```python
from build123d import *

# Parameters (mm, degrees)
F1_DEPTH = 25.4
F2_R     = 51.507819
F3_DEPTH = 203.2
F5_DEPTH = 25.4


with BuildPart() as f1:
    # F0 (on Front) → F1 (new body)
    with BuildSketch(Plane.XZ):
        Polygon((-28.796132, -69.520012), (28.796132, -69.520012), (69.520012, -28.796132), (69.520012, 28.796132), (28.796132, 69.520012), (-28.796132, 69.520012), (-69.520012, 28.796132), (-69.520012, -28.796132), align=None)
    extrude(amount=F1_DEPTH)

    # F2 (on Front) → F3 (join)
    with BuildSketch(Plane.XZ):
        Circle(F2_R)
    extrude(amount=F3_DEPTH)

    # F4 (on face) → F5 (join)
    with BuildSketch(Plane.XZ.offset(25.4)):
        Polygon((-28.796132, -69.520012), (28.796132, -69.520012), (69.520012, -28.796132), (69.520012, 28.796132), (28.796132, 69.520012), (-28.796132, 69.520012), (-69.520012, 28.796132), (-69.520012, -28.796132), align=None)
    extrude(amount=F5_DEPTH)


solid = f1.part
```
Geometry check sheet. Reference: the model listing, model coordinates, mm. A direction names the side the tool comes from. Coordinates: 2 decimals unless noted, no trailing zeros. Loops run counter-clockwise (first coordinate to the right, second up) from the corner with the lowest first, then second, coordinate; pieces in that order, holes last. Notation, with made-up numbers: (76, -20) - (133, -20) arc R13 cw to (133, -9) - close; hole circle Ø4 at (20.5, 65). An arc over 180 degrees is marked (long way). One line per item, written item: value. Start each with the question number.
(1) Depth check by flat-ended pin: P1, Ø5, axis at x = -44.5, y = -50.5, coming from the -Z side; P2, Ø2, axis at x = -47.5, z = -22.5, coming from the -Y side; P3, Ø1.5, axis at x = -45.5, y = -106.5, coming from the +Z side. Enter the tip coordinate at first touch or a pass-through.
(2) Cross-section at A-A on z = 0. Enter the section's corners in (x, y), plus the area to 3 significant figures.
(3) Cross-section at B-B on x = 0. Enter the section's corners in (y, z), plus the area to 3 significant figures.
(4) Cross-section at C-C on y = -99.5. Enter the section's corners in (x, z).
(5) Material ranges on line 1 (Z direction, x = 2, y = -150); line 2 (Y direction, x = -12, z = 51.5), recorded low to high. Write a range as [from, to].
(6) Tool access check on faces 1 (the flat face through (69.52, -25, 0)), 2 (the flat face through (-32, -50.8, 47)). Record the directions out of +Z, -Z, +X, -X, +Y, -Y that give a thin tool (end or side, any length) a straight path to the whole face; none if there is none.
Results below:
1. P1: stops at z = -56.32
1. P2: stops at y = -50.8
1. P3: stops at z = 25.5
2. outline: (-69.52, -50.8) - (-51.51, -50.8) - (-51.51, -203.2) - (51.51, -203.2) - (51.51, -50.8) - (69.52, -50.8) - (69.52, 0) - (-69.52, 0) - close
2. area: 22,800 mm2
3. outline: (-203.2, -51.51) - (-50.8, -51.51) - (-50.8, -69.52) - (0, -69.52) - (0, 69.52) - (-50.8, 69.52) - (-50.8, 51.51) - (-203.2, 51.51) - close
3. area: 22,800 mm2
4. outline: circle Ø103.02 at (0, 0)
5. line 1: z = [-51.47, 51.47]
5. line 2: y = [-50.8, 0]
6. face 1: +Z, -Z, +X, +Y, -Y
6. face 2: -Y
